Design review of the part built by this model. Coordinates are the model's own, in mm. A direction names the side the tool comes from. Coordinates: 2 decimals unless noted, no trailing zeros. Write each loop counter-clockwise with the first axis right and the second up, starting at its lowest first coordinate (ties: lowest second). Pieces come first, ordered by that corner, then holes.
Q1. Clearance check with flat-ended pins moving along their axes: pin 1 Ø8 at (x, z) = (-30, 22) entering from -Y; pin 2 Ø3.5 at (x, z) = (-33.02, -33.02) entering from -Y; pin 3 Ø6.5 at (x, z) = (33.02, 33.02) entering from +Y; pin 4 Ø5.5 at (x, z) = (8.5, 14.5) entering from +Y. State where each tip first meets the part, or that it passes through.
Q2. Add section A-A, the plane y = 10.5. Give the number of separate pieces and of enclosed holes in the cut face, plus the area to 3 significant figures.
Q3. Add section B-B, the plane x = 0. Give the boundary of the cut face in (y, z).
Q4. The part is to be moulded in two halves that separate along X. For faces 3 (the face through (12, 10, -21.589)), 4 (the face through (-38.1, 6, 0)), 5 (the face through (0, 6, 38.1)), 6 (the face through (3.555, 10, 13)), say which applies: +X half, -X half, draft (parallel to the pull), parting line (faces both ways), or undercut.
Q5. To check wall thickness, follow probe 1 along X at (y, z) = (3, 33.02); probe 2 along Z at (x, y) = (-16.5, 10.75). State the ranges of each line that lie inside material, in increasing order.
Q6. Machinability: for faces 1 (the face through (36.572, 6.439, -36.651)), 2 (the face through (-13, 10, 21.589)), which of the approach directions +Z, -Z, +X, -X, +Y, -Y give a long, thin tool a straight path to every point of the face, cutting with its end or side? Answer none if there is none.
from build123d import *

# Parameters (mm, degrees)
SKETCH1_W           = 76.2
SKETCH1_H           = 76.2
BOSS_EXTRUDE1_DEPTH = 12.7
SKETCH2_R           = 2.794
CUT_EXTRUDE1_DEPTH  = 56.358016583
SKETCH2_3_R         = 32.512
BOSS_EXTRUDE2_DEPTH = 5.08
SKETCH5_W           = 18.034
SKETCH5_H           = 18.034
CUT_EXTRUDE2_DEPTH  = 15.24
FILLET1_R           = 5.08
CHAMFER1_SIZE       = 1.778


with BuildPart() as part:
    # Sketch1 → Boss-Extrude1 (new body)
    with BuildSketch(Plane(origin=(0, 0, 0), x_dir=(1, 0, 0), z_dir=(0, 1, 0))):
        Rectangle(SKETCH1_W, SKETCH1_H)
    extrude(amount=BOSS_EXTRUDE1_DEPTH)

    # Sketch2 → Cut-Extrude1 (cut, through all)
    with BuildSketch(Plane(origin=(0, 12.7, 0), x_dir=(1, 0, 0), z_dir=(0, 1, 0))):
        with Locations(Location((33.02, 33.02, 0), (0, 0, 270))):
            Circle(SKETCH2_R)
        with Locations(Location((33.02, -33.02, 0), (0, 0, 270))):
            Circle(SKETCH2_R)
        with Locations(Location((-33.02, -33.02, 0), (0, 0, 270))):
            Circle(SKETCH2_R)
        with Locations(Location((-33.02, 33.02, 0), (0, 0, 270))):
            Circle(SKETCH2_R)
    extrude(amount=-CUT_EXTRUDE1_DEPTH, mode=Mode.SUBTRACT)

    # Sketch2_3 → Boss-Extrude2 (add)
    with BuildSketch(Plane(origin=(0, 12.7, 0), x_dir=(1, 0, 0), z_dir=(0, 1, 0))):
        with Locations(Location((0, 0, 0), (0, 0, 90))):
            Circle(SKETCH2_3_R)
    extrude(amount=BOSS_EXTRUDE2_DEPTH)

    # Sketch5 → Cut-Extrude2 (cut)
    with BuildSketch(Plane(origin=(0, 17.78, 0), x_dir=(1, 0, 0), z_dir=(0, 1, 0))):
        with Locations((-12.572358569, 12.572358569)):
            Rectangle(SKETCH5_W, SKETCH5_H)
        with Locations((12.572358569, 12.572358569)):
            Rectangle(SKETCH5_W, SKETCH5_H)
        with Locations((12.572358569, -12.572358569)):
            Rectangle(SKETCH5_W, SKETCH5_H)
        with Locations((-12.572358569, -12.572358569)):
            Rectangle(SKETCH5_W, SKETCH5_H)
    extrude(amount=-CUT_EXTRUDE2_DEPTH, mode=Mode.SUBTRACT)

    # Fillet1
    fillet1_edges = [part.edges().sort_by_distance(p)[0] for p in [
        (38.1, 6.35, 38.1),
        (-38.1, 6.35, 38.1),
        (-38.1, 6.35, -38.1),
        (38.1, 6.35, -38.1),
    ]]
    fillet(fillet1_edges, radius=FILLET1_R)

    # Chamfer1
    chamfer1_edges = [part.edges().sort_by_distance(p)[0] for p in [
        (0, 17.78, 32.512),
    ]]
    chamfer(chamfer1_edges, length=CHAMFER1_SIZE)


solid = part.part
Here are the results:
1. pin 1: stops at y = 0
1. pin 2: passes through
1. pin 3: stops at y = 12.7
1. pin 4: stops at y = 2.54
2. separate pieces: 1
2. enclosed holes: 8
2. area: 4,390 mm2
3. outline: (0, -38.1) - (12.7, -38.1) - (12.7, -32.51) - (16, -32.51) - (17.78, -30.73) - (17.78, 30.73) - (16, 32.51) - (12.7, 32.51) - (12.7, 38.1) - (0, 38.1) - close
4. face 3: undercut
4. face 4: -X half
4. face 5: draft
4. face 6: undercut
5. probe 1: x = -38.1 to -35.81, -30.23 to 30.23, 35.81 to 38.1
5. probe 2: z = -38.1 to -21.59, -3.56 to 3.56, 21.59 to 38.1
6. face 1: -Z, +X, +Y, -Y
6. face 2: +Y
